Design review of the part built by this model. Coordinates are the model's own, in mm. A direction names the side the tool comes from. Coordinates: 2 decimals unless noted, no trailing zeros. Write each loop counter-clockwise with the first axis right and the second up, starting at its lowest first coordinate (ties: lowest second). Pieces come first, ordered by that corner, then holes.
Q1. Take a section at A-A, the plane y = 234.5. Write out the cut boundary in (x, z).
Q2. For pin 1 Ø14.5 at (x, y) = (61.91, -68.58) entering from +Z (3 decimals); pin 2 Ø7 at (x, z) = (11, 2) entering from +Y; pin 3 Ø2 at (x, y) = (29, 641) entering from -Z; pin 4 Ø6 at (x, y) = (16, 910.5) entering from +Z, all flat-tipped, find the tip position at first contact; note any pin that passes through.
Q3. For L1, parallel to X at y = -21, z = 6; L2, parallel to Y at x = 63.5, z = 9.75; L3, parallel to Y at x = 70, z = 1.75, list the stretches that pass through material, from the lowest coordinate up.
Q4. The part is to be moulded in two halves that separate along X. For faces 4 (the flat face through (50.999, 835.117, 12.074)), 5 (the flat face through (12.88, 525.93, 9.57)), 6 (the flat face through (54, 222, 12.7)), say which applies: released by +X, released by -X, zero draft, split by the parting line, or undercut.
Q5. For faces 1 (the flat face through (51, 484, 11.43)), 2 (the flat face through (51, 832, 1.27)), 3 (the flat face through (54, 919, 12.7)), list the 3-axis set-ups (+Z, -Z, +X, -X, +Y, -Y) from which the entire face can be reached by the end or side of a thin tool; tool diameter is ignored.
Autodesk Inventor part; units mm, degrees
ref_plane "YZ Plane" through (0, 0, 0) normal (1, 0, 0) x (0, 1, 0)
ref_plane "XZ Plane" through (0, 0, 0) normal (0, 1, 0) x (-1, 0, 0)
ref_plane "XY Plane" through (0, 0, 0) normal (0, 0, 1) x (1, 0, 0)
sketch "Sketch1" plane through (0, 0, 0) normal (0, 0, 1) x (1, 0, 0)
  line L0 (0, 0) -> (82.55, 0)
  line L1 (82.55, 0) -> (82.55, 968.4207)
  line L2 (82.55, 968.4207) -> (82.55, 804.8513)
  line L3 (82.55, 804.8513) -> (82.55, 621.9713)
  line L4 (82.55, 621.9713) -> (82.55, 439.0913)
  line L5 (82.55, 439.0913) -> (82.55, 256.2113)
  line L6 (82.55, 256.2113) -> (82.55, 73.3313)
  line L7 (0, 1066.8) -> (0, 0)
  line L8 (0, 1066.8) -> (82.55, 968.4207)
  line L9 (-23.6845, 1095.0261) -> (784.1067, 132.338)
  line L10 (-109.2976, 1023.1881) -> (698.4936, 60.5001)
  line L11 (-194.9107, 951.3502) -> (612.8804, -11.3378)
  line L12 (-280.5239, 879.5122) -> (527.2673, -83.1758)
  line L13 (-366.137, 807.6743) -> (441.6542, -155.0137)
  line L14 (-451.7501, 735.8363) -> (356.041, -226.8517)
  dimension "d26" = 1066.8
  dimension "d27" = 82.55
  dimension "d28" = 40
  dimension "d34" = 111.76
  dimension "d35" = 111.76
  dimension "d36" = 111.76
  dimension "d37" = 111.76
  dimension "d38" = 111.76
extrude "Extrusion1" add sketch "Sketch1" along normal blind 12.7
sketch "Sketch2" plane through (0, 0, 12.7) normal (0, 0, 1) x (1, 0, 0)
  line L0 (0, 0) -> (82.55, 0)
  line L1 (82.55, 0) -> (82.55, 968.4207)
  line L2 (82.55, 968.4207) -> (82.55, 804.8513)
  line L3 (82.55, 804.8513) -> (82.55, 621.9713)
  line L4 (82.55, 621.9713) -> (82.55, 439.0913)
  line L5 (82.55, 439.0913) -> (82.55, 256.2113)
  line L6 (82.55, 256.2113) -> (82.55, 73.3313)
  line L7 (0, 1066.8) -> (0, 0)
  line L8 (0, 1066.8) -> (82.55, 968.4207)
  line L9 (-23.6845, 1095.0261) -> (784.1067, 132.338)
  line L10 (-109.2976, 1023.1881) -> (698.4936, 60.5001)
  line L11 (-194.9107, 951.3502) -> (612.8804, -11.3378)
  line L12 (-280.5239, 879.5122) -> (527.2673, -83.1758)
  line L13 (-366.137, 807.6743) -> (441.6542, -155.0137)
  line L14 (-451.7501, 735.8363) -> (356.041, -226.8517)
  line L15 (-453.2094, 734.6118) -> (354.5817, -228.0762)
  line L16 (-450.2908, 737.0609) -> (357.5004, -225.6272)
  line L17 (-367.5963, 806.4498) -> (440.1949, -156.2382)
  line L18 (-364.6777, 808.8988) -> (443.1135, -153.7892)
  line L19 (-281.9832, 878.2877) -> (525.808, -84.4003)
  line L20 (-279.0645, 880.7367) -> (528.7266, -81.9513)
  line L21 (-196.37, 950.1257) -> (611.4211, -12.5624)
  line L22 (-193.4514, 952.5747) -> (614.3397, -10.1133)
  line L23 (-110.7569, 1021.9636) -> (697.0342, 59.2756)
  line L24 (-107.8383, 1024.4126) -> (699.9529, 61.7246)
  point P0 (0, 889.9687)
  point P1 (82.55, 791.5894)
  point P2 (82.55, 797.5167)
  point P3 (0, 895.896)
  point P4 (0, 716.101)
  point P5 (82.55, 617.7217)
  point P6 (82.55, 623.649)
  point P7 (0, 722.0283)
  point P8 (0, 542.2333)
  point P9 (82.55, 443.854)
  point P10 (82.55, 449.7813)
  point P11 (0, 548.1606)
  point P12 (0, 368.3656)
  point P13 (82.55, 269.9863)
  point P14 (82.55, 275.9136)
  point P15 (0, 374.2929)
  point P16 (0, 194.4979)
  point P17 (82.55, 96.1186)
  point P18 (82.55, 102.0459)
  point P19 (0, 200.4252)
  dimension "d41" = 1066.8
  dimension "d42" = 82.55
  dimension "d43" = 40
  dimension "d44" = 111.76
  dimension "d45" = 111.76
  dimension "d46" = 111.76
  dimension "d47" = 111.76
  dimension "d48" = 111.76
  dimension "d49" = 1.905
  dimension "d50" = 1.905
  dimension "d51" = 1.905
  dimension "d52" = 1.905
  dimension "d53" = 1.905
  dimension "d54" = 1.905
  dimension "d55" = 1.905
  dimension "d56" = 1.905
  dimension "d57" = 1.905
  dimension "d58" = 1.905
extrude "Extrusion2" cut sketch "Sketch2" against normal blind 12.7 contours L7 L14 L1 L15 | L7 L16 L1 L14 | L7 L13 L1 L17 | L7 L18 L1 L13 | L7 L12 L1 L19 | L7 L20 L1 L12 | L7 L11 L1 L21 | L7 L22 L1 L11 | L7 L10 L1 L23 | L7 L24 L1 L10
sketch "Sketch3" plane through (0, 0, 12.7) normal (0, 0, 1) x (1, 0, 0)
  line L0 (0, 0) -> (82.55, 0)
  line L1 (82.55, 0) -> (82.55, 968.4207)
  line L2 (82.55, 968.4207) -> (82.55, 804.8513)
  line L3 (82.55, 804.8513) -> (82.55, 621.9713)
  line L4 (82.55, 621.9713) -> (82.55, 439.0913)
  line L5 (82.55, 439.0913) -> (82.55, 256.2113)
  line L6 (82.55, 256.2113) -> (82.55, 73.3313)
  line L7 (0, 1066.8) -> (0, 0)
  line L8 (0, 1066.8) -> (82.55, 968.4207)
  line L9 (-23.6845, 1095.0261) -> (784.1067, 132.338)
  line L10 (-109.2976, 1023.1881) -> (698.4936, 60.5001)
  line L11 (-194.9107, 951.3502) -> (612.8804, -11.3378)
  line L12 (-280.5239, 879.5122) -> (527.2673, -83.1758)
  line L13 (-366.137, 807.6743) -> (441.6542, -155.0137)
  line L14 (-451.7501, 735.8363) -> (356.041, -226.8517)
  line L15 (-453.2094, 734.6118) -> (354.5817, -228.0762)
  line L16 (-450.2908, 737.0609) -> (357.5004, -225.6272)
  line L17 (-367.5963, 806.4498) -> (440.1949, -156.2382)
  line L18 (-364.6777, 808.8988) -> (443.1135, -153.7892)
  line L19 (-281.9832, 878.2877) -> (525.808, -84.4003)
  line L20 (-279.0645, 880.7367) -> (528.7266, -81.9513)
  line L21 (-196.37, 950.1257) -> (611.4211, -12.5624)
  line L22 (-193.4514, 952.5747) -> (614.3397, -10.1133)
  line L23 (-110.7569, 1021.9636) -> (697.0342, 59.2756)
  line L24 (-107.8383, 1024.4126) -> (699.9529, 61.7246)
  point P0 (0, 889.9687)
  point P1 (82.55, 791.5894)
  point P2 (82.55, 797.5167)
  point P3 (0, 895.896)
  point P4 (0, 716.101)
  point P5 (82.55, 617.7217)
  point P6 (82.55, 623.649)
  point P7 (0, 722.0283)
  point P8 (0, 542.2333)
  point P9 (82.55, 443.854)
  point P10 (82.55, 449.7813)
  point P11 (0, 548.1606)
  point P12 (0, 368.3656)
  point P13 (82.55, 269.9863)
  point P14 (82.55, 275.9136)
  point P15 (0, 374.2929)
  point P16 (0, 194.4979)
  point P17 (82.55, 96.1186)
  point P18 (82.55, 102.0459)
  point P19 (0, 200.4252)
  point P20 (0, 889.9687)
  point P21 (82.55, 791.5894)
  point P22 (82.55, 797.5167)
  point P23 (0, 895.896)
  point P24 (0, 716.101)
  point P25 (82.55, 617.7217)
  point P26 (82.55, 623.649)
  point P27 (0, 722.0283)
  point P28 (0, 542.2333)
  point P29 (82.55, 443.854)
  point P30 (82.55, 449.7813)
  point P31 (0, 548.1606)
  point P32 (0, 368.3656)
  point P33 (82.55, 269.9863)
  point P34 (82.55, 275.9136)
  point P35 (0, 374.2929)
  point P36 (0, 194.4979)
  point P37 (82.55, 96.1186)
  point P38 (82.55, 102.0459)
  point P39 (0, 200.4252)
  dimension "d114" = 15.875
  dimension "d61" = 1066.8
  dimension "d62" = 82.55
  dimension "d63" = 40
  dimension "d64" = 111.76
  dimension "d65" = 111.76
  dimension "d66" = 111.76
  dimension "d67" = 111.76
  dimension "d68" = 111.76
  dimension "d69" = 1.905
  dimension "d70" = 1.905
  dimension "d71" = 1.905
  dimension "d72" = 1.905
  dimension "d73" = 1.905
  dimension "d74" = 1.905
  dimension "d75" = 1.905
  dimension "d76" = 1.905
  dimension "d77" = 1.905
  dimension "d78" = 1.905
extrude "Extrusion3" add sketch "Sketch3" against normal blind 11.43 contours L7 L14 L1 L15 | L7 L16 L1 L14 | L7 L13 L1 L17 | L7 L18 L1 L13 | L7 L12 L1 L19 | L7 L20 L1 L12 | L7 L11 L1 L21 | L7 L22 L1 L11 | L7 L10 L1 L23 | L7 L24 L1 L10
sketch "Sketch4" plane through (0, 0, 12.7) normal (0, 0, 1) x (1, 0, 0)
  line L0 (0, 0) -> (82.55, 0)
  line L1 (82.55, 0) -> (82.55, 968.4207)
  line L2 (82.55, 968.4207) -> (82.55, 804.8513)
  line L3 (82.55, 804.8513) -> (82.55, 621.9713)
  line L4 (82.55, 621.9713) -> (82.55, 439.0913)
  line L5 (82.55, 439.0913) -> (82.55, 256.2113)
  line L6 (82.55, 256.2113) -> (82.55, 73.3313)
  line L7 (0, 1066.8) -> (0, 0)
  line L8 (0, 1066.8) -> (82.55, 968.4207)
  line L9 (-23.6845, 1095.0261) -> (784.1067, 132.338)
  line L10 (-109.2976, 1023.1881) -> (698.4936, 60.5001)
  line L11 (-194.9107, 951.3502) -> (612.8804, -11.3378)
  line L12 (-280.5239, 879.5122) -> (527.2673, -83.1758)
  line L13 (-366.137, 807.6743) -> (441.6542, -155.0137)
  line L14 (-451.7501, 735.8363) -> (356.041, -226.8517)
  line L15 (-453.2094, 734.6118) -> (354.5817, -228.0762)
  line L16 (-450.2908, 737.0609) -> (357.5004, -225.6272)
  line L17 (-367.5963, 806.4498) -> (440.1949, -156.2382)
  line L18 (-364.6777, 808.8988) -> (443.1135, -153.7892)
  line L19 (-281.9832, 878.2877) -> (525.808, -84.4003)
  line L20 (-279.0645, 880.7367) -> (528.7266, -81.9513)
  line L21 (-196.37, 950.1257) -> (611.4211, -12.5624)
  line L22 (-193.4514, 952.5747) -> (614.3397, -10.1133)
  line L23 (-110.7569, 1021.9636) -> (697.0342, 59.2756)
  line L24 (-107.8383, 1024.4126) -> (699.9529, 61.7246)
  point P0 (0, 889.9687)
  point P1 (82.55, 791.5894)
  point P2 (82.55, 797.5167)
  point P3 (0, 895.896)
  point P4 (0, 716.101)
  point P5 (82.55, 617.7217)
  point P6 (82.55, 623.649)
  point P7 (0, 722.0283)
  point P8 (0, 542.2333)
  point P9 (82.55, 443.854)
  point P10 (82.55, 449.7813)
  point P11 (0, 548.1606)
  point P12 (0, 368.3656)
  point P13 (82.55, 269.9863)
  point P14 (82.55, 275.9136)
  point P15 (0, 374.2929)
  point P16 (0, 194.4979)
  point P17 (82.55, 96.1186)
  point P18 (82.55, 102.0459)
  point P19 (0, 200.4252)
  point P20 (0, 889.9687)
  point P21 (82.55, 791.5894)
  point P22 (82.55, 797.5167)
  point P23 (0, 895.896)
  point P24 (0, 716.101)
  point P25 (82.55, 617.7217)
  point P26 (82.55, 623.649)
  point P27 (0, 722.0283)
  point P28 (0, 542.2333)
  point P29 (82.55, 443.854)
  point P30 (82.55, 449.7813)
  point P31 (0, 548.1606)
  point P32 (0, 368.3656)
  point P33 (82.55, 269.9863)
  point P34 (82.55, 275.9136)
  point P35 (0, 374.2929)
  point P36 (0, 194.4979)
  point P37 (82.55, 96.1186)
  point P38 (82.55, 102.0459)
  point P39 (0, 200.4252)
  dimension "d81" = 1066.8
  dimension "d82" = 82.55
  dimension "d83" = 40
  dimension "d84" = 111.76
  dimension "d85" = 111.76
  dimension "d86" = 111.76
  dimension "d87" = 111.76
  dimension "d88" = 111.76
  dimension "d89" = 1.905
  dimension "d90" = 1.905
  dimension "d91" = 1.905
  dimension "d92" = 1.905
  dimension "d93" = 1.905
  dimension "d94" = 1.905
  dimension "d95" = 1.905
  dimension "d96" = 1.905
  dimension "d97" = 1.905
  dimension "d98" = 1.905
extrude "Extrusion4" cut sketch "Sketch4" against normal blind 1.27 contours L7 L14 L1 L15 | L7 L16 L1 L14 | L7 L13 L1 L17 | L7 L18 L1 L13 | L7 L12 L1 L19 | L7 L20 L1 L12 | L7 L11 L1 L21 | L7 L22 L1 L11 | L7 L10 L1 L23 | L7 L24 L1 L10
sketch "Sketch5" plane through (0, 0, 0) normal (0, -1, 0) x (1, 0, 0)
  line L0 (0, 12.7) -> (82.55, 12.7)
  line L1 (0, 12.7) -> (25.4, 12.7)
  line L2 (25.4, 12.7) -> (0, 6.35)
  line L3 (0, 0) -> (0, 12.7)
  line L4 (0, 6.35) -> (25.4, 0)
  line L5 (0, 0) -> (82.55, 0)
  dimension "d101" = 25.4
extrude "Extrusion5" cut sketch "Sketch5" against normal through all
sketch "Sketch6" plane through (0, 0, 12.7) normal (0, 0, 1) x (1, 0, 0)
  line L0 (25.4, 164.2273) -> (25.4, 0)
  line L1 (25.4, 0) -> (82.55, 0)
  line L2 (82.55, 0) -> (82.55, 96.1186)
  line L3 (82.55, 96.1186) -> (25.4, 164.2273)
  line L4 (0, 0) -> (82.55, 0)
  line L5 (82.55, 0) -> (82.55, -91.44)
  line L6 (82.55, -91.44) -> (0, -91.44)
  line L7 (0, -91.44) -> (0, 0)
  line L8 (0, -91.44) -> (45.72, -91.44)
  line L9 (45.72, -91.44) -> (45.72, -182.88)
  line L10 (82.55, -91.44) -> (45.72, -91.44)
  line L11 (45.72, -91.44) -> (45.72, -182.88)
  line L12 (45.72, -182.88) -> (82.55, -182.88)
  line L13 (82.55, -182.88) -> (82.55, -91.44)
  line L14 (0, -45.72) -> (82.55, -45.72)
  line L15 (25.4, 0) -> (82.55, 0)
  line L16 (41.275, 0) -> (41.275, -91.44)
  line L17 (45.72, -137.16) -> (82.55, -137.16)
  line L18 (0, -91.44) -> (0, -45.72)
  line L19 (0, -91.44) -> (41.275, -91.44)
  line L20 (41.275, -91.44) -> (82.55, -91.44)
  line L21 (82.55, -91.44) -> (82.55, -45.72)
  line L22 (82.55, -45.72) -> (82.55, 0)
  line L23 (82.55, 0) -> (41.275, 0)
  line L24 (25.4, 0) -> (0, 0)
  line L25 (41.275, 0) -> (0, 0)
  line L26 (82.55, -91.44) -> (82.55, -137.16)
  line L27 (45.72, -137.16) -> (45.72, -182.88)
  circle A0 centre (20.6375, -22.86) radius 7.9375
  circle A1 centre (61.9125, -22.86) radius 7.9375
  circle A2 centre (61.9125, -68.58) radius 7.9375
  circle A3 centre (20.6375, -68.58) radius 7.9375
  circle A4 centre (64.135, -114.3) radius 7.9375
  circle A5 centre (64.135, -160.02) radius 7.9375
  dimension "d104" = 91.44
  dimension "d106" = 91.44
  dimension "d107" = 45.72
  dimension "d108" = 91.44
  dimension "d109" = 36.83
  dimension "d110" = 15.875
  dimension "d111" = 15.875
  dimension "d112" = 15.875
  dimension "d113" = 15.875
  dimension "d114" = 15.875
  dimension "d115" = 15.875
extrude "Extrusion6" add sketch "Sketch6" against normal blind 12.7 contours L1 L16 L14 L7 L4 | L1 L5 L14 L16 | L16 L6 L7 L14 | L14 L5 L6 L16 | L13 L17 L9 L6 | L13 L12 L9 L17
properties part number "blade D 3.25"
Responses:
1. outline: (0, 6.35) - (25.4, 0) - (82.55, 0) - (82.55, 12.7) - (25.4, 12.7) - close
2. pin 1: passes through
2. pin 2: stops at y = 1056.87
2. pin 3: stops at z = 0
2. pin 4: stops at z = 11.1
3. L1: x = 0 to 12.92, 28.35 to 54.2, 69.63 to 82.55
3. L2: y = -182.88 to -167.93, -152.11 to -122.21, -106.39 to -76.36, -60.8 to -30.64, -15.08 to 991.12
3. L3: y = -182.88 to -165.37, -154.67 to -119.65, -108.95 to 983.38
4. face 4: undercut
4. face 5: released by -X
4. face 6: zero draft
5. face 1: +Z
5. face 2: -Z
5. face 3: +Z, +X, -X, +Y, -Y
